Input: part model. Units: mm. Frame: model coordinates. A direction names the side the tool comes from. Round coordinates to 2 decimals unless told otherwise and drop trailing zeros. Order: outer loops, then holes, each group sorted by start corner. A loop starts at its lowest first (then second) coordinate and runs counter-clockwise, first axis right, second up. Notation, with made-up numbers: M 3,75 L 32,75 A26 ccw 32,92 Z; hole C -20,15 d8. An arc over 180 degrees is marked long. One line per question, with ' | ' between items.
```python
from build123d import *

# Parameters (mm, degrees)
SKETCH1_W           = 25.4
SKETCH1_H           = 25.4
SKETCH1_W_2         = 22.352
SKETCH1_H_2         = 22.352
BOSS_EXTRUDE1_DEPTH = 25.4
SKETCH2_R           = 3.96875
SKETCH2_W           = 25.4
SKETCH2_H           = 12.7
CUT_EXTRUDE1_DEPTH  = 26.4
CUT_EXTRUDE2_DEPTH  = 26.4


with BuildPart() as part:
    # Sketch1 → Boss-Extrude1 (new body, symmetric)
    with BuildSketch(Plane.XY):
        Rectangle(SKETCH1_W, SKETCH1_H)
        Rectangle(SKETCH1_W_2, SKETCH1_H_2, mode=Mode.SUBTRACT)
    extrude(amount=BOSS_EXTRUDE1_DEPTH, both=True)

    # Sketch2 → Cut-Extrude1 (cut, through all)
    with BuildSketch(Plane(origin=(12.7, 0, 0), x_dir=(0, 0, -1), z_dir=(1, 0, 0))):
        with Locations((19.05, 0)):
            Circle(SKETCH2_R)
        with Locations((-9.525, 0)):
            Rectangle(SKETCH2_W, SKETCH2_H)
    extrude(amount=-CUT_EXTRUDE1_DEPTH, mode=Mode.SUBTRACT)

    # Sketch3 → Cut-Extrude2 (cut, through all)
    with BuildSketch(Plane(origin=(12.7, 0, 0), x_dir=(0, 0, -1), z_dir=(1, 0, 0))):
        Polygon((6.35, 12.7), (25.4, 6.35), (25.4, 12.7), align=None)
        Polygon((25.4, -6.35), (25.4, -12.7), (6.35, -12.7), align=None)
    extrude(amount=-CUT_EXTRUDE2_DEPTH, mode=Mode.SUBTRACT)


solid = part.part
```
Item 1: Section query D-D, the plane x = -4.5. Return loops of the section in (y, z).
Report:
outline: M -12.7,-6.35 L -11.18,-10.92 L -11.18,25.4 L -12.7,25.4 Z; M 11.18,-10.92 L 12.7,-6.35 L 12.7,25.4 L 11.18,25.4 Z
Item 2: Mould query, pull axis Y, two halves, no side actions, for faces 1 (the flat face through (-12.7, 0, -5)), 2 (the flat face through (-0.88, 11.42, -10.19)), 3 (the flat face through (11.176, 0, -5)). Classes: +Y half, -Y half, draft (parallel to the pull), parting line (faces both ways), or undercut.
Report:
face 1: draft | face 2: +Y half | face 3: undercut
Item 3: Access query for faces 4 (the flat face through (0, -12.7, 10)), 5 (the flat face through (-12, 0, -3.175)), 6 (the flat face through (0, 11.176, 7)). Directions: +Z, -Z, +X, -X, +Y, -Y. A direction counts if a zero-diameter tool reaches every point of the face in a straight line with its end or side. Return the directions, or none.
Report:
face 4: +Z, -Z, +X, -X, -Y | face 5: +X, -X | face 6: +Z, -Z
Item 4: Line query: line 1 along X through (y, z) = (6.5, -23); line 2 along Y through (x, z) = (-12.3, -19.05). Output: solid intervals per line, ascending. Write a range as from..to.
Report:
line 1: -12.7..-11.18, 11.18..12.7 | line 2: -8.47..-3.97, 3.97..8.47
Item 5: First-contact query: pin 1 (9 mm diameter, centred on y = 0, z = -19.05, fed in from -X); pin 2 (2 mm diameter, centred on x = 3, z = -9.5, fed in from +Y); pin 3 (7 mm diameter, centred on y = 0, z = -19.05, fed in from +X); pin 4 (2 mm diameter, centred on x = -0.5, z = -9.5, fed in from -Y). Flat tips, straight axial feed; report the tip coordinate or a pass-through.
Report:
pin 1: x = -12.7 | pin 2: y = 11.98 | pin 3: through | pin 4: y = -11.98
Item 6: Section query B-B, the plane y = 0. Return loops of the section in (x, z) (3 decimals), plus the area to 3 significant figures.
Report:
outline: M -12.7,-25.4 L -11.176,-25.4 L -11.176,-23.019 L -12.7,-23.019 Z; M -12.7,-15.081 L -11.176,-15.081 L -11.176,-3.175 L -12.7,-3.175 Z; M -12.7,22.225 L -11.176,22.225 L -11.176,25.4 L -12.7,25.4 Z; M 11.176,-25.4 L 12.7,-25.4 L 12.7,-23.019 L 11.176,-23.019 Z; M 11.176,-15.081 L 12.7,-15.081 L 12.7,-3.175 L 11.176,-3.175 Z; M 11.176,22.225 L 12.7,22.225 L 12.7,25.4 L 11.176,25.4 Z | area: 53.2 mm²
Item 7: Section query A-A, the plane y = 8. Return loops of the section in (x, z).
Report:
outline: M -12.7,-20.45 L -11.18,-20.45 L -11.18,25.4 L -12.7,25.4 Z; M 11.18,-20.45 L 12.7,-20.45 L 12.7,25.4 L 11.18,25.4 Z
Item 8: Section query C-C, the plane z = 20. Return loops of the section in (x, y).
Report:
outline: M -12.7,-12.7 L 12.7,-12.7 L 12.7,-6.35 L 11.18,-6.35 L 11.18,-11.18 L -11.18,-11.18 L -11.18,-6.35 L -12.7,-6.35 Z; M -12.7,6.35 L -11.18,6.35 L -11.18,11.18 L 11.18,11.18 L 11.18,6.35 L 12.7,6.35 L 12.7,12.7 L -12.7,12.7 Z
